```python
from build123d import *

# Parameters (mm, degrees)
SKETCH1_R           = 20
BOSS_EXTRUDE1_DEPTH = 2
SKETCH2_R           = 2
BOSS_EXTRUDE2_DEPTH = 1
SKETCH3_W           = 3
SKETCH3_H           = 20
BOSS_EXTRUDE3_DEPTH = 40
SKETCH5_R           = 1.5
CUT_EXTRUDE1_DEPTH  = 58.035076926


with BuildPart() as part:
    # Sketch1 → Boss-Extrude1 (new body)
    with BuildSketch(Plane.XY):
        Circle(SKETCH1_R)
    extrude(amount=BOSS_EXTRUDE1_DEPTH)

    # Sketch2 → Boss-Extrude2 (add)
    with BuildSketch(Plane(origin=(0, 0, 0), x_dir=(-1, 0, 0), z_dir=(0, 0, -1))):
        with Locations(Location((0, 0, 0), (0, 0, 180))):
            Circle(SKETCH2_R)
    extrude(amount=BOSS_EXTRUDE2_DEPTH)

    # Sketch3 → Boss-Extrude3 (add)
    with BuildSketch(Plane.XY.offset(2)):
        with Locations((-11.5, 0)):
            Rectangle(SKETCH3_W, SKETCH3_H)
    boss_extrude3 = extrude(amount=BOSS_EXTRUDE3_DEPTH)

    # Mirror1: Boss-Extrude3 across plane
    add(boss_extrude3.mirror(Plane(origin=(0, 0, 0), x_dir=(0, 0, 1), z_dir=(1, 0, 0))))

    # Sketch5 → Cut-Extrude1 (cut, through all)
    with BuildSketch(Plane.ZY.offset(13)):
        with Locations(Location((37, 0, 0), (0, 0, 270))):
            Circle(SKETCH5_R)
    extrude(amount=-CUT_EXTRUDE1_DEPTH, mode=Mode.SUBTRACT)


solid = part.part
```
Check sheet for the modelled part. Datum: model origin and axes. Units: mm. A direction names the side the tool comes from. Coordinates: 2 decimals unless noted, no trailing zeros. Write each loop counter-clockwise with the first axis right and the second up, starting at its lowest first coordinate (ties: lowest second). Pieces come first, ordered by that corner, then holes. Notation, with made-up numbers: M 40.25,1 L 86.25,1 A19 ccw 86.25,10 Z; hole C -13,54.25 d6. An arc over 180 degrees is marked long. Use one line per item in the form item = value.
Item 1: Sectioned sample at B-B, the plane z = 37. Record the cut outline in (x, y), and give its area (3 significant figures).
Answer below:
outline = M -13,-10 L -10,-10 L -10,-1.5 L -13,-1.5 Z; M -13,1.5 L -10,1.5 L -10,10 L -13,10 Z; M 10,-10 L 13,-10 L 13,-1.5 L 10,-1.5 Z; M 10,1.5 L 13,1.5 L 13,10 L 10,10 Z
area = 102 mm^2
Item 2: Release check for a two-part mould opening along Z. For faces 1 (the face through (12, 10, 22)), 2 (the face through (11.479, 0.325, 35.536)), 3 (the face through (4, 0, 0)) record: pulls with the +Z half, pulls with the -Z half, needs draft (parallel to the pull), parting line crosses it, or undercut.
Answer below:
face_1 = needs draft
face_2 = undercut
face_3 = pulls with the -Z half
Item 3: Set-up check for faces 4 (the face through (-10, 0, 22)), 5 (the face through (-12, -10, 22)), 6 (the face through (-0.434, 1.952, -0.493)), 7 (the face through (-12, 10, 22)): record each of +Z, -Z, +X, -X, +Y, -Y from which the full face is reachable in a straight line by a thin tool's end or side.
Answer below:
face_4 = +Z, +Y, -Y
face_5 = +Z, +X, -X, -Y
face_6 = -Z
face_7 = +Z, +X, -X, +Y
Item 4: Sectioned sample at C-C, the plane x = 0. Record the cut outline in (y, z), and give its area (3 significant figures).
Answer below:
outline = M -20,0 L -2,0 L -2,-1 L 2,-1 L 2,0 L 20,0 L 20,2 L -20,2 Z
area = 84.0 mm^2
Item 5: Sectioned sample at D-D, the plane z = 19.5. Record the cut outline in (x, y).
Answer below:
outline = M -13,-10 L -10,-10 L -10,10 L -13,10 Z; M 10,-10 L 13,-10 L 13,10 L 10,10 Z
Item 6: Gauge pin test, flat ends, axial feed: pin 1 Ø2.5 at (x, z) = (12, 27) entering from +Y; pin 2 Ø10 at (y, z) = (8.5, 31) entering from -X; pin 3 Ø4 at (x, y) = (-1.5, -9.5) entering from -Z; pin 4 Ø20 at (x, y) = (-7.5, -1) entering from +Z. Record the tip position at first contact, or that the pin passes through.
Answer below:
pin_1 = 10
pin_2 = -13
pin_3 = 0
pin_4 = 42
Item 7: Sectioned sample at A-A, the plane y = 0. Record the cut outline in (x, z), and give its area (3 significant figures).
Answer below:
outline = M -20,0 L -2,0 L -2,-1 L 2,-1 L 2,0 L 20,0 L 20,2 L 13,2 L 13,35.5 L 10,35.5 L 10,2 L -10,2 L -10,35.5 L -13,35.5 L -13,2 L -20,2 Z; M -13,38.5 L -10,38.5 L -10,42 L -13,42 Z; M 10,38.5 L 13,38.5 L 13,42 L 10,42 Z
area = 306 mm^2
Item 8: Material ranges on L1, parallel to X at y = -4, z = 13; L2, parallel to Z at x = 12, y = 0; L3, parallel to Z at x = -3, y = 15, recorded low to high. Write a range as from..to.
Answer below:
L1 = -13..-10, 10..13
L2 = 0..35.5, 38.5..42
L3 = 0..2
